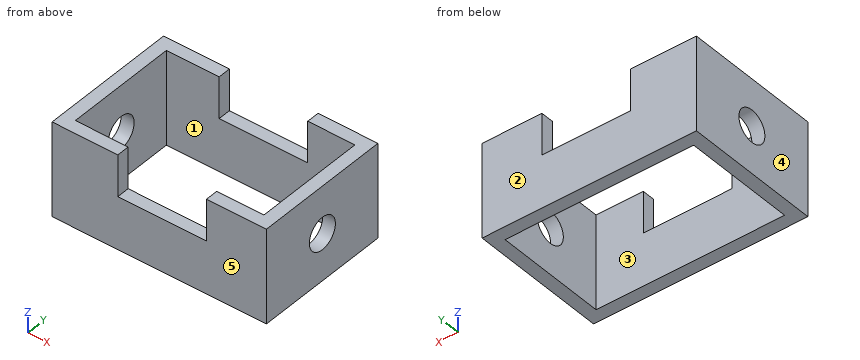
from build123d import *

# Parameters (mm, degrees)
F0_W     = 10.5373039842
F0_H     = 91.4049893618
F0_W_2   = 152.6683866978
F0_H_2   = 10.2922543883
F0_W_3   = 10.2922543883
F1_DEPTH = 76.2
F2_W     = 38.2388904691
F2_H     = 33.5443941772
F2_W_2   = 33.4795936942
F3_DEPTH = 111.9904981384
F4_R     = 13.0513622492
F5_DEPTH = 173.4989450703


with BuildPart() as f1:
    # F0 (on Top) → F1 (new body)
    with BuildSketch(Plane.XY):
        with Locations((-81.4803205431, -0.2450533211)):
            Rectangle(F0_W, F0_H)
        with Locations((0.1225247979, 50.6035685539)):
            Rectangle(F0_W_2, F0_H_2)
        with Locations((-81.4803205431, 50.6035685539)):
            Rectangle(F0_W, F0_H_2)
        with Locations((81.602845341, 50.6035685539)):
            Rectangle(F0_W_3, F0_H_2)
        with Locations((81.602845341, -0.2450533211)):
            Rectangle(F0_W_3, F0_H)
        with Locations((81.602845341, -51.0936751962)):
            Rectangle(F0_W_3, F0_H_2)
        with Locations((0.1225247979, -51.0936751962)):
            Rectangle(F0_W_2, F0_H_2)
        with Locations((-81.4803205431, -51.0936751962)):
            Rectangle(F0_W, F0_H_2)
    extrude(amount=F1_DEPTH)

    # F2 (on face) → F3 (cut, through all)
    with BuildSketch(Plane.XZ.offset(56.2398023903)):
        with Locations((19.1194452345, 59.4278029114)):
            Rectangle(F2_W, F2_H)
        with Locations((-16.7397968471, 59.4278029114)):
            Rectangle(F2_W_2, F2_H)
    extrude(amount=-F3_DEPTH, mode=Mode.SUBTRACT)

    # F4 (on face) → F5 (cut, through all)
    with BuildSketch(Plane.YZ.offset(86.7489725351)):
        with Locations((0, 38.1)):
            Circle(F4_R)
    extrude(amount=-F5_DEPTH, mode=Mode.SUBTRACT)


solid = f1.part
CAD build for the part. Positions are in the model's coordinates, mm. Face numbers are marked on the shaded views. A direction names the side the tool comes from. Round coordinates to 2 decimals unless told otherwise and drop trailing zeros. Write each loop counter-clockwise with the first axis right and the second up, starting at its lowest first coordinate (ties: lowest second). Pieces come first, ordered by that corner, then holes.
(1) Slice it at B-B, the plane x = 17. Write the cut outline in (y, z), and give its area (3 significant figures).
(2) Slice it at D-D, the plane y = -43. Write the cut outline in (x, z).
(3) Slice it at A-A, the plane z = 53. Write the cut outline in (x, y).
(4) Probe line 1 along Z through (x, y) = (79, 0); line 2 along X through (y, z) = (34.5, 69); line 3 along Y through (x, z) = (59, 68). List the from-to ranges inside material, lowest first.
(5) Mould opens along Y. For the marked faces 3, 4 and 5 say: pulls with the +Y half, pulls with the -Y half, needs draft (parallel to the pull), parting line crosses it, or undercut.
(6) Slice it at C-C, the plane y = 0. Write the cut outline in (x, z), and give its area (3 significant figures).
(7) Drop a flat-ended pin along its axis: P1, Ø8, axis at x = -13, y = -51.5, coming from the +Z side. Give the stop position or say it passes through.
(8) 3-axis set-ups, long thin cutter, end or side, ignore diameter. For the marked faces 1 and 2: which of +Z, -Z, +X, -X, +Y, -Y reach the whole face in a straight line?
From the geometry:
1. outline: (-56.24, 0) - (-45.95, 0) - (-45.95, 42.66) - (-56.24, 42.66) - close; (45.46, 0) - (55.75, 0) - (55.75, 42.66) - (45.46, 42.66) - close
1. area: 878 mm2
2. outline: (-86.75, 0) - (-76.21, 0) - (-76.21, 76.2) - (-86.75, 76.2) - close; (76.46, 0) - (86.75, 0) - (86.75, 76.2) - (76.46, 76.2) - close
3. outline: (-86.75, -56.24) - (-33.48, -56.24) - (-33.48, -45.95) - (-76.21, -45.95) - (-76.21, 45.46) - (-33.48, 45.46) - (-33.48, 55.75) - (-86.75, 55.75) - close; (38.24, -56.24) - (86.75, -56.24) - (86.75, 55.75) - (38.24, 55.75) - (38.24, 45.46) - (76.46, 45.46) - (76.46, -45.95) - (38.24, -45.95) - close
4. line 1: z = 0 to 25.05, 51.15 to 76.2
4. line 2: x = -86.75 to -76.21, 76.46 to 86.75
4. line 3: y = -56.24 to -45.95, 45.46 to 55.75
5. face 3: undercut
5. face 4: needs draft
5. face 5: pulls with the -Y half
6. outline: (-86.75, 0) - (-76.21, 0) - (-76.21, 25.05) - (-86.75, 25.05) - close; (-86.75, 51.15) - (-76.21, 51.15) - (-76.21, 76.2) - (-86.75, 76.2) - close; (76.46, 0) - (86.75, 0) - (86.75, 25.05) - (76.46, 25.05) - close; (76.46, 51.15) - (86.75, 51.15) - (86.75, 76.2) - (76.46, 76.2) - close
6. area: 1,040 mm2
7. P1: stops at z = 42.66
8. face 1: +Z, -Z
8. face 2: +Z, -Z, +X, -X, +Y
